Input: part model. Units: mm. Frame: model coordinates. A direction names the side the tool comes from. Coordinates: 2 decimals unless noted, no trailing zeros. Loops run counter-clockwise (first coordinate to the right, second up) from the corner with the lowest first, then second, coordinate; pieces in that order, holes last. Notation, with made-up numbers: (-24.75, 26.25) -> (7.25, 26.25) arc R11 ccw to (7.25, 30.25) -> close; hole circle Ø3 at (57.5, 19.5). An arc over 180 degrees is marked (long way). Put each result on its own line as item: value. Start each with the question number.
1) Cut plane A-A (x = 0). State how many separate pieces and enclosed holes the cut face has, plus the area to 3 significant figures.
2) Cut plane D-D (z = 20). Return the cut outline in (x, y), plus the area to 3 significant figures.
3) Material intervals for L1, parallel to X at y = 0.5, z = 20; L2, parallel to Y at x = 0, z = 19; L3, parallel to Z at x = 25.25, y = 0, sorted ascending.
4) Set-up query: faces 5 (the flat face through (32, 17, 23)), 6 (the flat face through (31.19, 7.51, 55.11)), 7 (the flat face through (-7.51, 31.19, 55.11)), 8 (the flat face through (-15.3, 0, 23)). Return all of +Z, -Z, +X, -X, +Y, -Y with unobstructed straight access to the full face (end or side cutting, diameter ignored); none if empty.
5) Cut plane C-C (z = 9). Return the cut outline in (x, y), plus the area to 3 significant figures.
6) Contact query for flat-ended pins moving along their axis: P1, Ø1, axis at x = 26, y = 13.5, coming from the +Z side; P2, Ø4.5, axis at x = -14, z = 11.5, coming from the +Y side; P3, Ø2, axis at x = 29.5, z = 43.5, coming from the -Y side. Output: stop coordinate, or through.
7) Pull-direction query (X, two-part tool) for faces 1 (the flat face through (-31.19, -7.51, 55.11)), 2 (the flat face through (7.42, 30.98, 55.11)), 3 (the flat face through (0, -34, 66)), 4 (the flat face through (-31.08, 7.19, 65.75)); classes: pulls with the +X half, pulls with the -X half, needs draft (parallel to the pull), parting line crosses it, or undercut.
from build123d import *

# Parameters (mm, degrees)
BOSS_EXTRUDE1_DEPTH = 21
CIRPATTERN1_COUNT   = 4
CHAMFER1_SIZE       = 0.5
SKETCH4_W           = 6.599999999999998
SKETCH4_H           = 8
CUT_EXTRUDE1_DEPTH  = 73.2841614740048
CHAMFER2_SIZE       = 0.5
FILLET1_R           = 1
CIRPATTERN4_COUNT   = 4


with BuildPart() as part:
    # Sketch1 → Revolve1 (revolve)
    with BuildSketch(Plane(origin=(0, 0, 0), x_dir=(0, 0, -1), z_dir=(1, 0, 0))):
        Polygon((-7.9e-16, 35), (0, 11.999999999999998), (-45, 11.999999999999995), (-45, 39.999999999999986), (-23, 39.99999999999999), (-23, 35), align=None)
    revolve(axis=Axis((0, 0, 0), (0, -1.2e-16, 1)))

    # Sketch3 → Boss-Extrude1 (add)
    with BuildSketch(Plane.XY.offset(44.99999999999999)):
        with BuildLine():
            ThreePointArc((-4.365000000000001, 23.599719807658744), (-2.1916574340201906, 23.89972045217066), (-3.535e-13, 24.00000000000001))
            Line((0, 24.00000000000001), (0, 40))
            ThreePointArc((1.49969e-12, 40), (-5.332266542852567, 39.642993498422584), (-10.569350394509474, 38.578346675798365))
            Line((-10.569350394509476, 38.57834667579836), (-4.365, 23.599719807658744))
        make_face()
        with BuildLine():
            Line((0, 40), (0, 24.00000000000001))
            ThreePointArc((-3.5261e-13, 24.00000000000001), (2.191657434019837, 23.89972045217069), (4.365, 23.599719807658744))
            Line((4.365, 23.599719807658744), (10.569350394509485, 38.57834667579835))
            ThreePointArc((10.569350394509485, 38.57834667579835), (5.332266542854057, 39.64299349842238), (1.49969e-12, 40))
        make_face()
    boss_extrude1 = extrude(amount=BOSS_EXTRUDE1_DEPTH)

    # CirPattern1: Boss-Extrude1 ×4 about axis
    cirpattern1_axis = Axis((6e-17, -4.97e-15, 0), (0, 0, 1))
    for i in range(1, CIRPATTERN1_COUNT):
        add(boss_extrude1.rotate(cirpattern1_axis, i * 360 / CIRPATTERN1_COUNT))

    # Chamfer1
    chamfer1_edges = [part.edges().sort_by_distance(p)[0] for p in [
        (4.4e-16, 24.000000000000004, 66),
        (-7.467175197254738, 31.089033241728544, 66),
        (7.467175197254742, 31.08903324172854, 66),
        (9.77e-15, 39.999999999999986, 66),
        (24.000000000000007, -1.068e-14, 66),
        (31.08903324172855, 7.467175197254726, 66),
        (31.089033241728547, -7.467175197254755, 66),
        (39.99999999999999, -2.356e-14, 66),
        (-3.26e-15, -24.000000000000014, 66),
        (7.467175197254734, -31.089033241728554, 66),
        (-7.467175197254746, -31.08903324172855, 66),
        (-1.455e-14, -39.99999999999999, 66),
        (-24.000000000000007, -1.92e-15, 66),
        (-31.08903324172855, -7.46717519725474, 66),
        (-31.089033241728547, 7.467175197254741, 66),
        (-39.99999999999999, 9.18e-15, 66),
    ]]
    chamfer(chamfer1_edges, length=CHAMFER1_SIZE)

    # Sketch4 → Cut-Extrude1 (cut, through all)
    with BuildSketch(Plane.XY.offset(44.99999999999999)):
        with Locations((-12.000000000000002, 0)):
            Rectangle(SKETCH4_W, SKETCH4_H)
    extrude(amount=-CUT_EXTRUDE1_DEPTH, mode=Mode.SUBTRACT)

    # Chamfer2
    chamfer2_edges = [part.edges().sort_by_distance(p)[0] for p in [
        (-4.9e-15, -39.99999999999999, 22.999999999999993),
        (-4.29e-15, -35, -7.95e-15),
    ]]
    chamfer(chamfer2_edges, length=CHAMFER2_SIZE)

    # Fillet1
    fillet1_edges = [part.edges().sort_by_distance(p)[0] for p in [
        (-4.29e-15, -35, 22.999999999999993),
    ]]
    fillet(fillet1_edges, radius=FILLET1_R)

    # Sketch6 → M8x1.25 Tapped Hole1 (revolve, cut)
    with BuildSketch(Plane(origin=(0, 0, 10), x_dir=(0, 0, 1), z_dir=(0, 1, 0))):
        Polygon((0, 0), (-9.8e-15, 39.99999999999999), (3.3999999999999946, 39.99999999999999), (3.3999999999999995, 3.6e-16), align=None)
    m8x1_25_tapped_hole1 = revolve(axis=Axis((-6.349999999999991, 0, 10), (1, 0, 0)), mode=Mode.SUBTRACT)

    # CirPattern4: M8x1.25 Tapped Hole1 ×4 about axis, 2 skipped
    cirpattern4_axis = Axis((0, 0, 0), (0, -1.2e-16, 1))
    add([m8x1_25_tapped_hole1.rotate(cirpattern4_axis, i * 360 / CIRPATTERN4_COUNT) for i in range(1, CIRPATTERN4_COUNT) if i not in (1, 2)], mode=Mode.SUBTRACT)


solid = part.part
Results found:
1. separate pieces: 3
1. enclosed holes: 0
1. area: 2,810 mm2
2. outline: circle Ø70 at (0, 0); hole (-15.3, -4) -> (-11.31, -4) arc R12 ccw (long way) to (-11.31, 4) -> (-15.3, 4) -> close
2. area: 3,370 mm2
3. L1: x = -35 to -15.3, 11.99 to 35
3. L2: y = -35 to -12, 12 to 35
3. L3: z = 0 to 6.6, 13.4 to 66
4. face 5: -Z
4. face 6: +Z, +Y
4. face 7: +Z, -X
4. face 8: +Z, -Z
5. outline: (-15.3, -4) -> (-15.3, 4) -> (-11.31, 4) arc R12 cw to (11.55, 3.25) -> (34.85, 3.25) arc R35 ccw (long way) to (-3.25, -34.85) -> (-3.25, -11.55) arc R12 cw to (-11.31, -4) -> close; (3.25, -34.85) arc R35 ccw to (34.85, -3.25) -> (11.55, -3.25) arc R12 cw to (3.25, -11.55) -> close
5. area: 3,070 mm2
6. P1: stops at z = 45
6. P2: stops at y = 32.97
6. P3: stops at y = -28.07
7. face 1: undercut
7. face 2: pulls with the +X half
7. face 3: needs draft
7. face 4: undercut
